Read the model definition and answer for the solid it produces. Units are mm, in the model's axes. A direction names the side the tool comes from. Round coordinates to 2 decimals unless told otherwise and drop trailing zeros. Loops run counter-clockwise (first coordinate to the right, second up) from the corner with the lowest first, then second, coordinate; pieces in that order, holes last. Notation, with made-up numbers: M -35.5,68.25 L -14.5,68.25 A29 cw -14.5,96.25 Z; hole C -32.75,63 d4. An arc over 180 degrees is marked long. Answer as CSV lines item,"result".
```python
from build123d import *

# Parameters (mm, degrees)
BOSS_EXTRU_1_DEPTH   = 10.3
ESQUISSE3_W          = 7.85
ESQUISSE3_H          = 20.6
ESQUISSE3_R          = 2.2
BOSS_EXTRU_2_DEPTH   = 2.8
BOSS_EXTRU_3_DEPTH   = 0.6
ESQUISSE8_R          = 6.1
BOSS_EXTRU_7_DEPTH   = 0.5
ESQUISSE5_R          = 2.925
BOSS_EXTRU_4_DEPTH   = 3.9
CONG_1_R             = 2
ESQUISSE6_W          = 3
ESQUISSE6_H          = 6.8
BOSS_EXTRU_5_DEPTH   = 5.3
ESQUISSE7_R          = 0.75
BOSS_EXTRU_6_DEPTH   = 5.3
D_GAGEMENT_M31_D     = 3.2
D_GAGEMENT_M31_DEPTH = 6
D_GAGEMENT_M31_TIP   = 0.96137699
CONG_2_R             = 1.6


with BuildPart() as part:
    # Esquisse1 → Boss.-Extru.1 (new, symmetric)
    with BuildSketch(Plane(origin=(0, 0, 0), x_dir=(1, 0, 0), z_dir=(0, 1, 0))):
        Polygon((-20.25, 12.5), (14.25, 12.5), (18.25, 8.5), (20.25, 8.5), (20.25, -24.7), (-20.25, -24.7), align=None)
    extrude(amount=BOSS_EXTRU_1_DEPTH, both=True)

    # Esquisse3 → Boss.-Extru.2 (add)
    # profile 1 of 2: a face of its own
    with BuildSketch(Plane.XY):
        with Locations((24.175, 0)):
            Rectangle(ESQUISSE3_W, ESQUISSE3_H)
        with Locations((24.5, 5)):
            Circle(ESQUISSE3_R, mode=Mode.SUBTRACT)
        with Locations(Location((24.5, -5, 0), (0, 0, 180))):
            Circle(ESQUISSE3_R, mode=Mode.SUBTRACT)
    # profile 2 of 2: a face of its own
    with BuildSketch(Plane.XY):
        with Locations((-24.175, 0)):
            Rectangle(ESQUISSE3_W, ESQUISSE3_H)
        with Locations(Location((-24.5, 5, 0), (0, 0, 180))):
            Circle(ESQUISSE3_R, mode=Mode.SUBTRACT)
        with Locations((-24.5, -5)):
            Circle(ESQUISSE3_R, mode=Mode.SUBTRACT)
    extrude(amount=-BOSS_EXTRU_2_DEPTH)

    # Esquisse4 → Boss.-Extru.3 (add, symmetric)
    with BuildSketch(Plane(origin=(0, 0, 0), x_dir=(1, 0, 0), z_dir=(0, 1, 0))):
        Polygon((20.25, 2.8), (20.25, 3.8), (23.75, 2.8), align=None)
        Polygon((-23.75, 2.8), (-20.25, 3.8), (-20.25, 2.8), align=None)
    extrude(amount=BOSS_EXTRU_3_DEPTH, both=True)

    # Esquisse8 → Boss.-Extru.7 (add)
    with BuildSketch(Plane(origin=(0, 0, -12.5), x_dir=(-1, 0, 0), z_dir=(0, 0, -1))):
        with Locations(Location((10.25, 0, 0), (0, 0, 180))):
            Circle(ESQUISSE8_R)
    extrude(amount=BOSS_EXTRU_7_DEPTH)

    # Esquisse5 → Boss.-Extru.4 (add)
    with BuildSketch(Plane(origin=(0, 0, -13), x_dir=(-1, 0, 0), z_dir=(0, 0, -1))):
        with Locations((10, 0)):
            Circle(ESQUISSE5_R)
    extrude(amount=BOSS_EXTRU_4_DEPTH)

    # Congé1
    cong_1_edges = [part.edges().sort_by_distance(p)[0] for p in [
        (28.1, 10.3, -1.4),
        (28.1, -10.3, -1.4),
        (-28.1, -10.3, -1.4),
        (-28.1, 10.3, -1.4),
    ]]
    fillet(cong_1_edges, radius=CONG_1_R)

    # Esquisse6 → Boss.-Extru.5 (add)
    with BuildSketch(Plane.ZY.offset(20.25)):
        with Locations((20.2, 0)):
            Rectangle(ESQUISSE6_W, ESQUISSE6_H)
    extrude(amount=BOSS_EXTRU_5_DEPTH)

    # Esquisse7 → Boss.-Extru.6 (add)
    with BuildSketch(Plane.ZY.offset(25.55)):
        with Locations((20.2, 0)):
            Circle(ESQUISSE7_R)
        with Locations((20.2, 1.6)):
            Circle(ESQUISSE7_R)
        with Locations(Location((20.2, -1.6, 0), (0, 0, 180))):
            Circle(ESQUISSE7_R)
    extrude(amount=BOSS_EXTRU_6_DEPTH)

    # Dégagement M31
    with Locations(Plane(origin=(0, 0, -16.9), x_dir=(-1, 0, 0), z_dir=(0, 0, -1))):
        with Locations((10, 0)):
            Hole(D_GAGEMENT_M31_D / 2, depth=D_GAGEMENT_M31_DEPTH)
            with Locations((0, 0, -(D_GAGEMENT_M31_DEPTH + D_GAGEMENT_M31_TIP / 2))):  # 118° drill point
                Cone(0, D_GAGEMENT_M31_D / 2, D_GAGEMENT_M31_TIP, mode=Mode.SUBTRACT)

    # Congé2
    cong_2_edges = [part.edges().sort_by_distance(p)[0] for p in [
        (-20.25, 0, -12.5),
    ]]
    fillet(cong_2_edges, radius=CONG_2_R)


solid = part.part
```
1) Find section B-B, the plane y = 5. Give the vertices of the cut face in (x, z), then the cut area to 3 significant figures.
Evaluation:
outline,"M -28.1,-2.8 L -26.7,-2.8 L -26.7,0 L -28.1,0 Z; M -22.3,-2.8 L -20.25,-2.8 L -20.25,-10.9 A1.6 ccw -18.65,-12.5 L -13.74,-12.5 L -13.74,-13 L -6.76,-13 L -6.76,-12.5 L 14.25,-12.5 L 18.25,-8.5 L 20.25,-8.5 L 20.25,-2.8 L 22.3,-2.8 L 22.3,0 L 20.25,0 L 20.25,24.7 L -20.25,24.7 L -20.25,0 L -22.3,0 Z; M 26.7,-2.8 L 28.1,-2.8 L 28.1,0 L 26.7,0 Z"
area,"1,510 mm^2"
2) Determine the mould class of faces 6 (the flat face through (-30.85, 0, 20)), 7 (the cylindrical face through (-28.163, 0.225, 20.915)), 8 (the flat face through (0, 10.3, 6)) for opening direction Y: released by +Y, released by -Y, zero draft, split by the parting line, or undercut.
Evaluation:
face 6,"zero draft"
face 7,"undercut"
face 8,"released by +Y"
3) Find section D-D, the plane x = 16. Give the vertices of the cut face in (y, z).
Evaluation:
outline,"M -10.3,-10.75 L 10.3,-10.75 L 10.3,24.7 L -10.3,24.7 Z"
4) Straight lines are drawn through the part: line 1 (Y direction, x = 24.5, z = -1.3); line 2 (Y direction, x = -24, z = -1); line 3 (Z direction, x = 21, y = -5.75). For each, find the intervals that lie inside material, in ascending order.
Evaluation:
line 1,"y = -10.3 to -7.2, -2.8 to 2.8, 7.2 to 10.3"
line 2,"y = -10.3 to -7.14, -2.86 to 2.86, 7.14 to 10.3"
line 3,"z = -2.8 to 0"
5) Find section A-A, the plane x = -24.5. Give the vertices of the cut face in (y, z), then the cut area to 3 significant figures.
Evaluation:
outline,"M -10.3,-2.8 L -7.2,-2.8 L -7.2,0 L -10.3,0 Z; M -3.4,18.7 L 3.4,18.7 L 3.4,21.7 L -3.4,21.7 Z; M -2.8,-2.8 L 2.8,-2.8 L 2.8,0 L -2.8,0 Z; M 7.2,-2.8 L 10.3,-2.8 L 10.3,0 L 7.2,0 Z"
area,"53.4 mm^2"
6) A tool of negligible diameter and unlimited length cuts with its end or side. For faces 1 (the flat face through (-25.55, 1, 21)), 2 (the cylindrical face through (-7.078, 0.129, -14.923)), 3 (the flat face through (24, 0, -2.8)), 4 (the flat face through (-23, 3.4, 20)), 5 (the flat face through (-23, 0, 18.7)), from which of +Z, -Z, +X, -X, +Y, -Y can it reach the whole face along a straight path? Write none if from no direction.
Evaluation:
face 1,"-X"
face 2,"-Z"
face 3,"-Z, +X"
face 4,"+Z, -X, +Y"
face 5,"-X, +Y, -Y"
7) Find section C-C, the plane z = 20.2. Give the vertices of the cut face in (x, y).
Evaluation:
outline,"M -30.85,-2.35 L -25.55,-2.35 L -25.55,-3.4 L -20.25,-3.4 L -20.25,-10.3 L 20.25,-10.3 L 20.25,10.3 L -20.25,10.3 L -20.25,3.4 L -25.55,3.4 L -25.55,2.35 L -30.85,2.35 L -30.85,0.85 L -25.55,0.85 L -25.55,0.75 L -30.85,0.75 L -30.85,-0.75 L -25.55,-0.75 L -25.55,-0.85 L -30.85,-0.85 Z"
8) Each of these flat-tipped pins is pushed along its axis until it touches: P1, Ø1.5, axis at x = 5, y = 0, coming from the -Z side; P2, Ø8, axis at y = -1.5, z = 16.5, coming from the +X side; P3, Ø2.5, axis at x = -24.5, y = -5, coming from the -Z side; P4, Ø3, axis at x = -10, y = 0, coming from the -Z side. Where does it stop, or does it pass through?
Evaluation:
P1,"stops at z = -12.5"
P2,"stops at x = 20.25"
P3,"passes through"
P4,"stops at z = -10.84"
